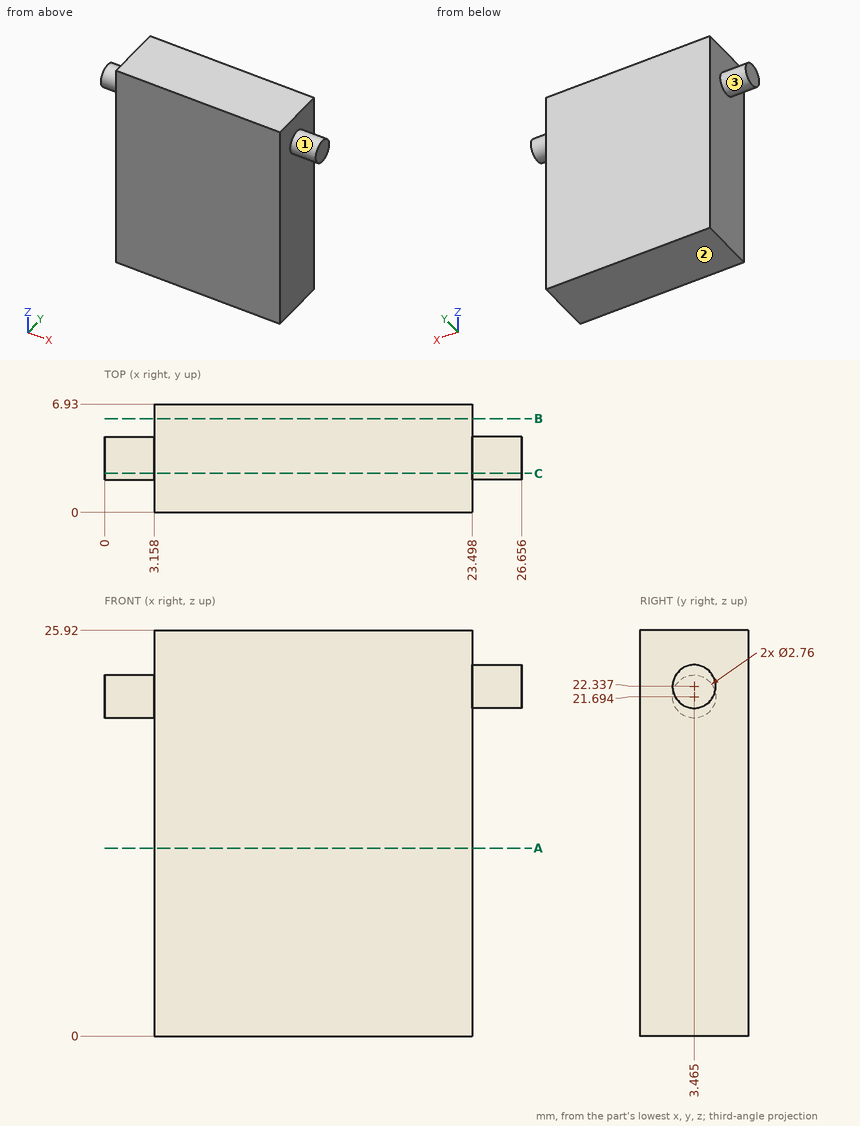
For this review, use the dimensioned drawing (mm, ordinates from the lowest corner) and the shaded views. A direction names the side the tool comes from. Give positions to 0.01 mm unless a question says otherwise; leave off trailing zeros. Loops run counter-clockwise (first coordinate to the right, second up) from the corner with the lowest first, then second, coordinate; pieces in that order, holes last. Notation, with made-up numbers: (63.25, 42.5) - (80.25, 42.5) arc R34 ccw to (80.25, 75.5) - close; hole circle Ø9 at (-36, 42). An arc over 180 degrees is marked (long way). Write each question's results on one line, items separated by ' | '.
(1) For line 1 along X through (y, z) = (4.5, 20.5), list the stretches that pass through material, from the lowest coordinate up.
Conclusion:
line 1: 3.16 to 23.5
(2) Take a section at C-C (y = 2.5). Give the boundary of the cut face in (x, z), then the cut area to 3 significant figures.
Conclusion:
outline: (0, 20.71) - (3.16, 20.71) - (3.16, 0) - (23.5, 0) - (23.5, 21.35) - (26.66, 21.35) - (26.66, 23.32) - (23.5, 23.32) - (23.5, 25.92) - (3.16, 25.92) - (3.16, 22.68) - (0, 22.68) - close | area: 540 mm^2
(3) Take a section at A-A (z = 12). Give the boundary of the cut face in (x, y).
Conclusion:
outline: (3.16, 0) - (23.5, 0) - (23.5, 6.93) - (3.16, 6.93) - close
(4) For the marked faces 1, 2 and 3, list the 3-axis set-ups (+Z, -Z, +X, -X, +Y, -Y) from which the entire face can be reached by the end or side of a thin tool; tool diameter is ignored.
Conclusion:
face 1: +X | face 2: -Z, +X, -X, +Y, -Y | face 3: -X
(5) For pin 1 Ø5 at (x, z) = (17.5, 12) entering from -Y; pin 2 Ø2 at (y, z) = (5.5, 14) entering from -X, all flat-tipped, find the tip position at first contact; note any pin that passes through.
Conclusion:
pin 1: y = 0 | pin 2: x = 3.16
(6) Take a section at B-B (y = 6). Give the boundary of the cut face in (x, z).
Conclusion:
outline: (3.16, 0) - (23.5, 0) - (23.5, 25.92) - (3.16, 25.92) - close
